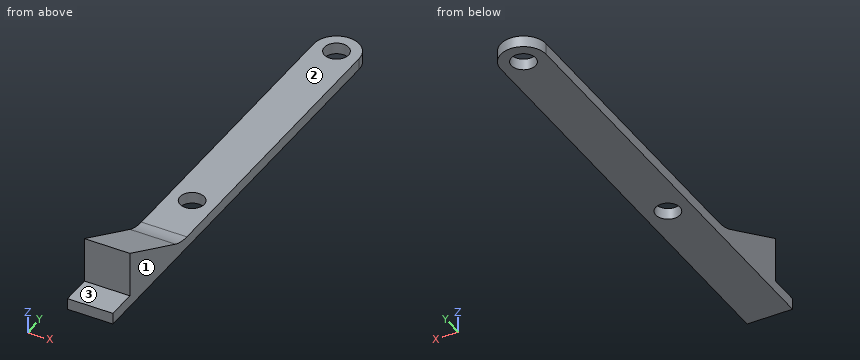
```python
from build123d import *

# Parameters (mm, degrees)
SKETCH_R     = 1.6
PAD_DEPTH    = 1.5
PAD001_DEPTH = 6
FILLET_R     = 6


with BuildPart() as part:
    # Sketch → Pad (new body)
    with BuildSketch(Plane.XY):
        with BuildLine():
            ThreePointArc((3, 16.999999), (-7e-06, 20), (-3, 16.999986))
            Line((-3, 16.999986), (-3, -37))
            Line((-3, -37), (-3, -41))
            Line((-3, -41), (3, -41))
            Line((3, -41), (3, -36.999987))
            Line((3, -36.999987), (3, 16.999999))
        make_face()
        with Locations((0, 17)):
            Circle(SKETCH_R, mode=Mode.SUBTRACT)
        with Locations((0, -17)):
            Circle(SKETCH_R, mode=Mode.SUBTRACT)
    extrude(amount=PAD_DEPTH)

    # Sketch001 → Pad001 (new body)
    with BuildSketch(Plane(origin=(-3, 0, 0), x_dir=(0, -1, 0), z_dir=(-1, 0, 0))):
        Polygon((37, 0), (37, 7.5), (22, 0), align=None)
    extrude(amount=-PAD001_DEPTH)

    # Fillet
    fillet_edges = [part.edges().sort_by_distance(p)[0] for p in [
        (0, -25, 1.5),
    ]]
    fillet(fillet_edges, radius=FILLET_R)


solid = part.part
```
Geometry: final body of the model. Coordinates: model frame, mm. Face numbers are marked on the shaded views. A direction names the side the tool comes from. Round coordinates to 2 decimals unless told otherwise and drop trailing zeros. Order: outer loops, then holes, each group sorted by start corner. A loop starts at its lowest first (then second) coordinate and runs counter-clockwise, first axis right, second up. Notation, with made-up numbers: (31, 50.25) -> (52, 50.25) arc R11 ccw to (52, 68.25) -> close; hole circle Ø5 at (29.25, 22.5). An arc over 180 degrees is marked (long way). Use CSV: the item, a comma, the result in double quotes. Start each with the question number.
1) First-contact query: pin 1 Ø3 at (x, z) = (1.5, 4) entering from -Y; pin 2 Ø3 at (x, y) = (-1, -12) entering from +Z. Flat tips, straight axial feed; report the tip coordinate or a pass-through.
2) Section B-B (y = -17). Return the cut outline in (x, z).
3) Section A-A (x = 0). Return the cut outline in (y, z), and give its area (3 significant figures).
4) Section D-D (x = 2.25). Return the cut outline in (y, z).
5) Set-up query: the marked faces 1, 2 and 3. Return all of +Z, -Z, +X, -X, +Y, -Y with unobstructed straight access to the full face (end or side cutting, diameter ignored); none if empty.
6) Material intervals for line 1 along Y through (x, z) = (0, 1.1); line 2 along Z through (x, y) = (2.25, -0.5); line 3 along Y through (x, z) = (-2.5, 6.75), sorted ascending. Write a range as from..to.
7) Section C-C (z = 6.25). Return the cut outline in (x, y), and give its area (3 significant figures).
Returned:
1,pin 1,"stops at y = -37"
1,pin 2,"stops at z = 1.5"
2,outline,"(-3, 0) -> (-1.6, 0) -> (-1.6, 1.5) -> (-3, 1.5) -> close; (1.6, 0) -> (3, 0) -> (3, 1.5) -> (1.6, 1.5) -> close"
3,outline,"(-41, 0) -> (-18.6, 0) -> (-18.6, 1.5) -> (-23.58, 1.5) arc R6 cw to (-26.27, 2.13) -> (-37, 7.5) -> (-37, 1.5) -> (-41, 1.5) -> close; (-15.4, 0) -> (15.4, 0) -> (15.4, 1.5) -> (-15.4, 1.5) -> close; (18.6, 0) -> (20, 0) -> (20, 1.5) -> (18.6, 1.5) -> close"
3,area,"118 mm²"
4,outline,"(-41, 0) -> (18.98, 0) -> (18.98, 1.5) -> (-23.58, 1.5) arc R6 cw to (-26.27, 2.13) -> (-37, 7.5) -> (-37, 1.5) -> (-41, 1.5) -> close"
5,face 1,"+Z, -Z, +X, +Y, -Y"
5,face 2,"+Z, +X, -X, +Y"
5,face 3,"+Z, +X, -X, -Y"
6,line 1,"y = -41..-18.6, -15.4..15.4, 18.6..20"
6,line 2,"z = 0..1.5"
6,line 3,"y = -37..-35.5"
7,outline,"(-3, -37) -> (3, -37) -> (3, -34.5) -> (-3, -34.5) -> close"
7,area,"15.0 mm²"
